Geometry check sheet. Reference: the model listing, model coordinates, mm. A direction names the side the tool comes from. Coordinates: 2 decimals unless noted, no trailing zeros. Write each loop counter-clockwise with the first axis right and the second up, starting at its lowest first coordinate (ties: lowest second). Pieces come first, ordered by that corner, then holes. Notation, with made-up numbers: M 50.25,4 L 76.25,4 A22 cw 76.25,33 Z; hole C 71.25,22 d9. An arc over 180 degrees is marked long. Write each question's results on one line, items separated by ' | '.
```python
from build123d import *

# Parameters (mm, degrees)
SKETCH1_W           = 25
SKETCH1_H           = 20
BOSS_EXTRUDE1_DEPTH = 8
FILLET1_R           = 1
SKETCH5_R           = 1.15
CUT_EXTRUDE1_DEPTH  = 5


with BuildPart() as part:
    # Sketch1 → Boss-Extrude1 (new body)
    with BuildSketch(Plane(origin=(0, 0, 0), x_dir=(1, 0, 0), z_dir=(0, 1, 0))):
        Rectangle(SKETCH1_W, SKETCH1_H)
    extrude(amount=BOSS_EXTRUDE1_DEPTH)

    # Sketch4 → CBORE for M3 SHCS1 (revolve, cut)
    with BuildSketch(Plane(origin=(-5, 8, 0), x_dir=(0, 0, 1), z_dir=(1, 0, 0))):
        Polygon((0, 0), (0, 8), (1.7, 8), (1.7, 3), (3.25, 3), (3.25, 0.025), (3.275, 0), align=None)
    revolve(axis=Axis((-5, 14.35, 0), (0, -1, 0)), mode=Mode.SUBTRACT)

    # Fillet1
    fillet1_edges = [part.edges().sort_by_distance(p)[0] for p in [
        (-12.5, 4, -10),
        (12.5, 4, -10),
        (12.5, 4, 10),
        (-12.5, 4, 10),
    ]]
    fillet(fillet1_edges, radius=FILLET1_R)

    # Sketch5 → Cut-Extrude1 (cut)
    with BuildSketch(Plane(origin=(0, 8, 0), x_dir=(1, 0, 0), z_dir=(0, 1, 0))):
        with Locations((4.5, 5)):
            Circle(SKETCH5_R)
        with Locations((4.5, -4.5)):
            Circle(SKETCH5_R)
    extrude(amount=-CUT_EXTRUDE1_DEPTH, mode=Mode.SUBTRACT)


solid = part.part
```
Q1. Mould release check, pull along Z, two halves, no side actions. Record for faces 1 (the flat face through (0, 4, 10)), 2 (the flat face through (-3.6, 5, -1.4)), 3 (the cylindrical face through (12.199, 4.056, -9.715)), 4 (the flat face through (-12.5, 4, 0)): pulls with the +Z half, pulls with the -Z half, needs draft (parallel to the pull), parting line crosses it, or undercut.
Geometry check:
face 1: pulls with the +Z half | face 2: undercut | face 3: pulls with the -Z half | face 4: needs draft
Q2. Sectioned sample at B-B on x = -5. Record the cut outline in (y, z) (3 decimals), and give its area (3 significant figures).
Geometry check:
outline: M 0,-10 L 8,-10 L 8,-3.275 L 7.975,-3.25 L 5,-3.25 L 5,-1.7 L 0,-1.7 Z; M 0,1.7 L 5,1.7 L 5,3.25 L 7.975,3.25 L 8,3.275 L 8,10 L 0,10 Z | area: 123 mm2
Q3. Sectioned sample at A-A on y = 1.5. Record the cut outline in (x, z).
Geometry check:
outline: M -12.5,-9 A1 ccw -11.5,-10 L 11.5,-10 A1 ccw 12.5,-9 L 12.5,9 A1 ccw 11.5,10 L -11.5,10 A1 ccw -12.5,9 Z; hole C -5,0 d3.4
Q4. Sectioned sample at C-C on z = 0. Record the cut outline in (x, y) (3 decimals).
Geometry check:
outline: M -12.5,0 L -6.7,0 L -6.7,5 L -8.25,5 L -8.25,7.975 L -8.275,8 L -12.5,8 Z; M -3.3,0 L 12.5,0 L 12.5,8 L -1.725,8 L -1.75,7.975 L -1.75,5 L -3.3,5 Z
Q5. Depth check by flat-ended pin: P1, Ø2.5, axis at x = 5, z = 4.5, coming from the +Y side; P2, Ø0.7, axis at x = 4, z = -5.5, coming from the +Y side; P3, Ø2.5, axis at x = -5, z = 0, coming from the -Y side. Enter the tip coordinate at first touch or a pass-through.
Geometry check:
P1: stops at y = 8 | P2: stops at y = 3 | P3: passes through
Q6. Access from +Z, -Z, +X, -X, +Y, -Y to the whole of each face (thin tool, end or side, straight path). Record for faces 5 (the flat face through (12.5, 4, 0)), 6 (the flat face through (4, 3, -5)).
Geometry check:
face 5: +Z, -Z, +X, +Y, -Y | face 6: +Y
Q7. Scan lines: probe 1 along Z at (x, y) = (4.5, 4.85); probe 2 along Z at (x, y) = (-5, 1.05); probe 3 along X at (y, z) = (3.15, 0). Record each from-to range of solid material in increasing order.
Geometry check:
probe 1: z = -10 to -6.15, -3.85 to 3.35, 5.65 to 10 | probe 2: z = -10 to -1.7, 1.7 to 10 | probe 3: x = -12.5 to -6.7, -3.3 to 12.5
Q8. Sectioned sample at D-D on y = 7. Record the cut outline in (x, z).
Geometry check:
outline: M -12.5,-9 A1 ccw -11.5,-10 L 11.5,-10 A1 ccw 12.5,-9 L 12.5,9 A1 ccw 11.5,10 L -11.5,10 A1 ccw -12.5,9 Z; hole C -5,0 d6.5; hole C 4.5,-5 d2.3; hole C 4.5,4.5 d2.3
